Source: CAD feature listing. Evaluate the final solid. Frame: model axes, mm. Coordinates: 2 decimals unless noted, no trailing zeros. Order: outer loops, then holes, each group sorted by start corner. A loop starts at its lowest first (then second) coordinate and runs counter-clockwise, first axis right, second up. Notation, with made-up numbers: (-2, 17.25) -> (56, 17.25) arc R10 cw to (56, 36.25) -> close; hole circle Ø1 at (4.25, 68). An arc over 180 degrees is marked (long way). Write item = value, one per line. Start each with the question number.
Item 1: Ray query, line 1 along Z through (x, y) = (0, 6.25); line 2 along X through (y, z) = (2, -57). Return the intervals inside material, ascending. Write a range as [from, to].
Item 2: Mould query, pull axis Z, two halves, no side actions, for faces 1 (the flat face through (1, 0, 1)), 2 (the cylindrical face through (0.365, 4.93, -62.276)), 3 (the cylindrical face through (48, 5, 74)), 4 (the cylindrical face through (-1.51, 4.93, 57.14)). Classes: released by +Z, released by -Z, zero draft, split by the parting line, or undercut.
Item 3: Contact query for a flat-ended pin moving along its axis: pin 1 (4.5 mm diameter, centred on x = 0, z = -59.5, fed in from -Y). Output: stop coordinate, or through.
Item 4: Section query A-A (z = 59.5). Output: boundary loops of the cut face in (x, y).
Item 5: Section query B-B (x = 0). Output: boundary loops of the cut face in (y, z), then the cut area to 3 significant figures.
Autodesk Inventor part; units mm, degrees
ref_plane "YZ Plane" through (0, 0, 0) normal (1, 0, 0) x (0, 1, 0)
ref_plane "XZ Plane" through (0, 0, 0) normal (0, 1, 0) x (-1, 0, 0)
ref_plane "XY Plane" through (0, 0, 0) normal (0, 0, 1) x (1, 0, 0)
sketch "Sketch1" plane through (0, 0, 0) normal (0, 1, 0) x (-1, 0, 0)
  line L0 (50, 75) -> (-50, 75)
  line L1 (-50, 75) -> (-50, -75)
  line L2 (-50, -75) -> (50, -75)
  line L3 (50, -75) -> (50, 75)
  line L4 (50, 75) -> (-50, -75) construction
  line L5 (-50, 75) -> (50, -75) construction
  circle A0 centre (0, 59.5) radius 2.8
  line L6 (0, 0) -> (50, 0) construction
  circle A1 centre (0, -59.5) radius 2.8
  dimension "d0" = 150
  dimension "d1" = 100
  dimension "d2" = 59.5
  dimension "d3" = 5.6
extrude "Extrusion1" add sketch "Sketch1" along normal blind 10
fillet "Fillet1" radius 5 4 edges at (50, 5, 75) (50, 5, -75) (-50, 5, 75) (-50, 5, -75)
properties part number "Base"
Computed:
q1.line_1 = [-75, -62.3], [-56.7, 56.7], [62.3, 75]
q1.line_2 = [-50, -1.26], [1.26, 50]
q2.face_1 = zero draft
q2.face_2 = undercut
q2.face_3 = released by +Z
q2.face_4 = undercut
q3.pin_1 = through
q4.outline = (-50, 0) -> (-2.8, 0) -> (-2.8, 10) -> (-50, 10) -> close; (2.8, 0) -> (50, 0) -> (50, 10) -> (2.8, 10) -> close
q5.outline = (0, -75) -> (10, -75) -> (10, -62.3) -> (0, -62.3) -> close; (0, -56.7) -> (10, -56.7) -> (10, 56.7) -> (0, 56.7) -> close; (0, 62.3) -> (10, 62.3) -> (10, 75) -> (0, 75) -> close
q5.area = 1,390 mm^2
